```python
from build123d import *

# Parameters (mm, degrees)
BOSS_EXTRUDE1_DEPTH        = 3
M3_CLEARANCE_HOLE1_D       = 3.242
F_3_5_3_5_DIAMETER_HOLE1_D = 3.5
SKETCH14_R                 = 11.075
CUT_EXTRUDE1_DEPTH         = 50.404579747
SKETCHED_START             = 0.899268265
SKETCHED_BEND1_OUTLINE_W   = 3
SKETCHED_BEND1_OUTLINE_H   = 42.5
SKETCHED_BEND1_DEPTH       = 15.700731735
SKETCHED_START_2           = -1.484291735
SKETCHED_BEND1_2_OUTLINE_R = 1.621
SKETCHED_BEND1_2_DEPTH     = 0.01644
SKETCHED_START_3           = -4.484291735
SKETCHED_BEND1_3_OUTLINE_R = 1.621
SKETCHED_BEND1_3_DEPTH     = 6
SKETCHED_START_4           = -21.25
SKETCHED_BEND1_4_DEPTH     = 42.5


with BuildPart() as part:
    # Sketch7 → Boss-Extrude1 (new body)
    with BuildSketch(Plane(origin=(0, 0, 0), x_dir=(1, 0, 0), z_dir=(0, 1, 0))):
        with BuildLine():
            Line((-40.5, -21.25), (10.6, -21.25))
            ThreePointArc((10.6, -21.25), (14.842640687, -19.492640687), (16.6, -15.25))
            Line((16.6, -15.25), (16.6, 15.25))
            ThreePointArc((16.6, 15.25), (14.842640687, 19.492640687), (10.6, 21.25))
            Line((10.6, 21.25), (-40.5, 21.25))
            Line((-40.5, 21.25), (-44.5, 17.25))
            Line((-44.5, 17.25), (-44.5, -17.25))
            Line((-44.5, -17.25), (-40.5, -21.25))
        make_face()
    extrude(amount=-BOSS_EXTRUDE1_DEPTH)

    # M3 Clearance Hole1 (through all)
    with Locations(Plane(origin=(0, -3, 0), x_dir=(-1, 0, 0), z_dir=(0, -1, 0))):
        with Locations((-9.084084573, -12.5), (-9.084084573, 12.5)):
            Hole(M3_CLEARANCE_HOLE1_D / 2)

    # Ø3.5 (3.5) Diameter Hole1 (through all)
    with Locations(Plane(origin=(0, 0, 0), x_dir=(1, 0, 0), z_dir=(0, 1, 0))):
        with Locations((-7.5, -15.5), (-38.5, -15.5), (-38.5, 15.5), (-7.5, 15.5)):
            Hole(F_3_5_3_5_DIAMETER_HOLE1_D / 2)

    # Sketch14 → Cut-Extrude1 (cut, through all)
    with BuildSketch(Plane.XZ.offset(3)):
        with Locations(Location((-23, 0, 0), (0, 0, 90))):
            Circle(SKETCH14_R)
    extrude(amount=-CUT_EXTRUDE1_DEPTH, mode=Mode.SUBTRACT)

    # Sketched Bend1: read off the stored shape, not the designer's step
    # Sketched Bend1 outline → Sketched Bend1 (cut)
    with BuildSketch(Plane.YZ.offset(SKETCHED_START)):
        with Locations((-1.5, 0)):
            Rectangle(SKETCHED_BEND1_OUTLINE_W, SKETCHED_BEND1_OUTLINE_H)
    extrude(amount=SKETCHED_BEND1_DEPTH, mode=Mode.SUBTRACT)

    # Sketched Bend1 2 outline → Sketched Bend1 2 (add)
    with BuildSketch(Plane.YZ.offset(SKETCHED_START_2)):
        with BuildLine():
            Line((0, -21.25), (11.015708265, -21.25))
            ThreePointArc((11.015708265, -21.25), (15.258348952, -19.492640687), (17.015708265, -15.25))
            Line((17.015708265, -15.25), (17.015708265, 15.25))
            ThreePointArc((17.015708265, 15.25), (15.258348952, 19.492640687), (11.015708265, 21.25))
            Line((11.015708265, 21.25), (0, 21.25))
            Line((0, 21.25), (0, -21.25))
        make_face()
        with Locations((9.499792838, -12.5)):
            Circle(SKETCHED_BEND1_2_OUTLINE_R, mode=Mode.SUBTRACT)
        with Locations((9.499792838, 12.5)):
            Circle(SKETCHED_BEND1_2_OUTLINE_R, mode=Mode.SUBTRACT)
    extrude(amount=SKETCHED_BEND1_2_DEPTH)

    # Sketched Bend1 3 outline → Sketched Bend1 3 (add)
    with BuildSketch(Plane.YZ.offset(SKETCHED_START_3)):
        with BuildLine():
            Line((0, -21.25), (11.015708265, -21.25))
            ThreePointArc((11.015708265, -21.25), (15.258348952, -19.492640687), (17.015708265, -15.25))
            Line((17.015708265, -15.25), (17.015708265, 15.25))
            ThreePointArc((17.015708265, 15.25), (15.258348952, 19.492640687), (11.015708265, 21.25))
            Line((11.015708265, 21.25), (0, 21.25))
            Line((0, 21.25), (0, -21.25))
        make_face()
        with Locations((9.499792838, -12.5)):
            Circle(SKETCHED_BEND1_3_OUTLINE_R, mode=Mode.SUBTRACT)
        with Locations((9.499792838, 12.5)):
            Circle(SKETCHED_BEND1_3_OUTLINE_R, mode=Mode.SUBTRACT)
    extrude(amount=SKETCHED_BEND1_3_DEPTH)

    # Sketched Bend1 4 outline → Sketched Bend1 4 (cut)
    with BuildSketch(Plane.XY.offset(SKETCHED_START_4)):
        with BuildLine():
            Line((-1.484291735, 3), (-1.484291735, 17.015708265))
            Line((-1.484291735, 17.015708265), (-4.484291735, 17.015708265))
            Line((-4.484291735, 17.015708265), (-4.484291735, 0))
            ThreePointArc((-4.484291735, 0), (-2.362971392, 0.878679656), (-1.484291735, 3))
        make_face()
        with BuildLine():
            Line((1.515708265, 0), (1.515708265, 3))
            ThreePointArc((1.515708265, 3), (-0.241651048, -1.242640687), (-4.484291735, -3))
            Line((-4.484291735, -3), (0.899268265, -3))
            Line((0.899268265, -3), (0.899268265, 0))
            Line((0.899268265, 0), (1.515708265, 0))
        make_face()
    extrude(amount=SKETCHED_BEND1_4_DEPTH, mode=Mode.SUBTRACT)


solid = part.part
```
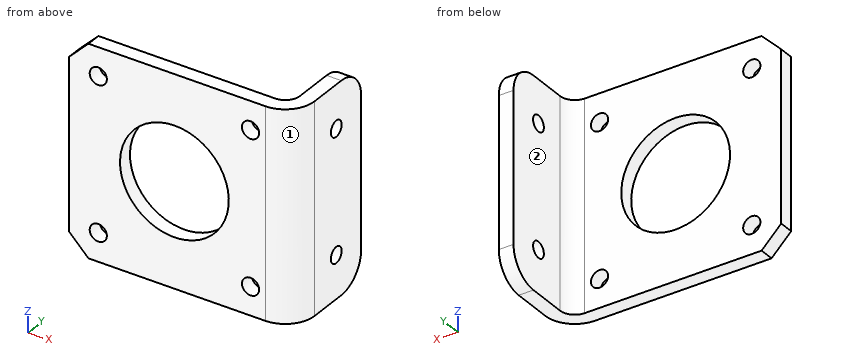
Here's how the part is built. I have some questions about the finished solid (model axes, mm). Face numbers are marked on the shaded views. A direction names the side the tool comes from. Round coordinates to 2 decimals unless told otherwise and drop trailing zeros. Order: outer loops, then holes, each group sorted by start corner. A loop starts at its lowest first (then second) coordinate and runs counter-clockwise, first axis right, second up. Notation, with made-up numbers: (2, 35.5) -> (43, 35.5) arc R14 ccw to (43, 41.5) -> close; hole circle Ø7 at (-32, -27.75). An arc over 180 degrees is marked (long way). Use a Markdown table: item, result. Add a question column.
(1) For the marked faces 1 and 2, which set-ups out of +Z, -Z, +X, -X, +Y, -Y let a thin tool reach every point of the face, with its end or its side?
(2) I need wall thicknesses on line 1 along Z through (x, y) = (-38.5, -0.7); line 2 along X through (y, z) = (-2.15, -15.5); line 3 along X through (y, z) = (-2.35, -15.5). Which ranges of each line are inside material? Lowest first, please.
(3) Suppose I cut it at D-D, the plane x = -38.5. Please give me the cut outline in (y, z).
(4) Suppose I cut it at C-C, the plane y = 9.25. Please give me the cut outline in (x, z), and give its area (3 significant figures).
(5) For pin 1 Ø4 at (y, z) = (12, 8.5) entering from -X; pin 2 Ø5 at (x, z) = (-38.5, 10.5) entering from +Y; pin 3 Ø4.5 at (x, z) = (-38.5, 15.5) entering from -Y, each with a flat end and sliding along its axis, tell me the tip position at first contact or that it passes through.
(6) Suppose I cut it at B-B, the plane x = -23. Please give me the cut outline in (y, z) (3 decimals).
(7) Suppose I cut it at A-A, the plane z = 0. Please give me the cut outline in (x, y) (3 decimals), and give its area (3 significant figures).
Verdict:
| question | item | result |
|---|---|---|
| 1 | face 1 | +Z, -Z, +X, -Y |
| 1 | face 2 | +Z, -Z, -X, +Y |
| 2 | line 1 | -21.25 to -17.25, -13.75 to 13.75, 17.25 to 21.25 |
| 2 | line 2 | -44.5 to -40.25, -36.75 to -9.25, -5.75 to -1.41 |
| 2 | line 3 | -44.5 to -40.25, -36.75 to -9.25, -5.75 to -1.77 |
| 3 | outline | (-3, -21.25) -> (0, -21.25) -> (0, -17.25) -> (-3, -17.25) -> close; (-3, -13.75) -> (0, -13.75) -> (0, 13.75) -> (-3, 13.75) -> close; (-3, 17.25) -> (0, 17.25) -> (0, 21.25) -> (-3, 21.25) -> close |
| 4 | outline | (-1.48, -21.25) -> (1.52, -21.25) -> (1.52, -14.1) -> (-1.48, -14.1) -> close; (-1.48, -10.9) -> (1.52, -10.9) -> (1.52, 10.9) -> (-1.48, 10.9) -> close; (-1.48, 14.1) -> (1.52, 14.1) -> (1.52, 21.25) -> (-1.48, 21.25) -> close |
| 4 | area | 108 mm2 |
| 5 | pin 1 | x = -1.48 |
| 5 | pin 2 | y = 0 |
| 5 | pin 3 | y = -3 |
| 6 | outline | (-3, -21.25) -> (0, -21.25) -> (0, -11.075) -> (-3, -11.075) -> close; (-3, 11.075) -> (0, 11.075) -> (0, 21.25) -> (-3, 21.25) -> close |
| 7 | outline | (-44.5, -3) -> (-34.075, -3) -> (-34.075, 0) -> (-44.5, 0) -> close; (-11.925, -3) -> (-4.484, -3) arc R6 ccw to (1.516, 3) -> (1.516, 17.016) -> (-1.484, 17.016) -> (-1.484, 3) arc R3 cw to (-4.484, 0) -> (-11.925, 0) -> close |
| 7 | area | 117 mm2 |
